Autodesk Inventor part; units mm, degrees
ref_plane "YZ Plane" through (0, 0, 0) normal (1, 0, 0) x (0, 1, 0)
ref_plane "XZ Plane" through (0, 0, 0) normal (0, 1, 0) x (-1, 0, 0)
ref_plane "XY Plane" through (0, 0, 0) normal (0, 0, 1) x (1, 0, 0)
sketch "Sketch1" plane through (0, 0, 0) normal (0, 0, 1) x (1, 0, 0)
  circle A0 centre (0, 0) radius 203.2
  dimension "d0" = 406.4
extrude "Extrusion1" add sketch "Sketch1" along normal blind 50.8
sketch "Sketch2" plane through (0, 0, 0) normal (1, 0, 0) x (0, 1, 0)
  circle A0 centre (-285.75, 25.4) radius 88.9
  line L0 (203.2, 0) -> (-203.2, 0)
  line L1 (0, 149.86) -> (0, -99.06)
  point P0 (0, 0)
  dimension "d3" = 25.4
  dimension "d4" = 177.8
  dimension "d5" = 285.75
revolve "Revolution1" cut sketch "Sketch2" angle 360 about axis through (0, 0, 0) along (0, 0, -1)
sketch "Sketch3" plane through (0, 0, 0) normal (0, 0, -1) x (-1, 0, 0)
  point P0 (0, 0)
sketch "Sketch4" plane through (0, 0, 50.8) normal (0, 0, 1) x (1, 0, 0)
  line L0 (-3.6662, 6.35) -> (3.6662, 6.35)
  line L1 (3.6662, 6.35) -> (7.3323, 0)
  line L2 (7.3323, 0) -> (3.6662, -6.35)
  line L3 (3.6662, -6.35) -> (-3.6662, -6.35)
  line L4 (-3.6662, -6.35) -> (-7.3323, 0)
  line L5 (-7.3323, 0) -> (-3.6662, 6.35)
  circle A0 centre (0, 23.8125) radius 2.5797
  circle A1 centre (-11.9062, 20.6222) radius 2.5797
  circle A2 centre (-20.6222, 11.9063) radius 2.5797
  circle A3 centre (-23.8125, 0) radius 2.5797
  circle A4 centre (-20.6222, -11.9062) radius 2.5797
  circle A5 centre (-11.9063, -20.6222) radius 2.5797
  circle A6 centre (0, -23.8125) radius 2.5797
  circle A7 centre (11.9062, -20.6222) radius 2.5797
  circle A8 centre (20.6222, -11.9063) radius 2.5797
  circle A9 centre (23.8125, 0) radius 2.5797
  circle A10 centre (20.6222, 11.9062) radius 2.5797
  circle A11 centre (11.9063, 20.6222) radius 2.5797
  point P0 (0, 0)
  point P1 (0, 0)
  dimension "d7" = 12.7
  dimension "d8" = 23.8125
  dimension "d9" = 5.1594
  dimension "d12" = 360
extrude "Extrusion2" cut sketch "Sketch4" against normal through all
sketch "Sketch6" plane through (0, 0, 0) normal (0, 0, -1) x (-1, 0, 0)
  circle A0 centre (0, 107.95) radius 2.5797
  circle A1 centre (0, 120.269) radius 4.445
  circle A2 centre (-41.3107, 99.7328) radius 2.5797
  circle A3 centre (-46.025, 111.1141) radius 4.445
  circle A4 centre (-76.3322, 76.3322) radius 2.5797
  circle A5 centre (-85.043, 85.043) radius 4.445
  circle A6 centre (-99.7328, 41.3107) radius 2.5797
  circle A7 centre (-111.1141, 46.025) radius 4.445
  circle A8 centre (-107.95, 0) radius 2.5797
  circle A9 centre (-120.269, 0) radius 4.445
  circle A10 centre (-99.7328, -41.3107) radius 2.5797
  circle A11 centre (-111.1141, -46.025) radius 4.445
  circle A12 centre (-76.3322, -76.3322) radius 2.5797
  circle A13 centre (-85.043, -85.043) radius 4.445
  circle A14 centre (-41.3107, -99.7328) radius 2.5797
  circle A15 centre (-46.025, -111.1141) radius 4.445
  circle A16 centre (0, -107.95) radius 2.5797
  circle A17 centre (0, -120.269) radius 4.445
  circle A18 centre (41.3107, -99.7328) radius 2.5797
  circle A19 centre (46.025, -111.1141) radius 4.445
  circle A20 centre (76.3322, -76.3322) radius 2.5797
  circle A21 centre (85.043, -85.043) radius 4.445
  circle A22 centre (99.7328, -41.3107) radius 2.5797
  circle A23 centre (111.1141, -46.025) radius 4.445
  circle A24 centre (107.95, 0) radius 2.5797
  circle A25 centre (120.269, 0) radius 4.445
  circle A26 centre (99.7328, 41.3107) radius 2.5797
  circle A27 centre (111.1141, 46.025) radius 4.445
  circle A28 centre (76.3322, 76.3322) radius 2.5797
  circle A29 centre (85.043, 85.043) radius 4.445
  circle A30 centre (41.3107, 99.7328) radius 2.5797
  circle A31 centre (46.025, 111.1141) radius 4.445
  point P0 (0, 0)
  dimension "d16" = 5.1594
  dimension "d17" = 107.95
  dimension "d18" = 8.89
  dimension "d19" = 120.269
  dimension "d22" = 360
extrude "Extrusion3" cut sketch "Sketch6" against normal through all
sketch "Sketch7" plane through (0, 0, 50.8) normal (0, 0, 1) x (1, 0, 0)
  circle A0 centre (0, 63.4238) radius 2.032
  circle A1 centre (-44.8474, 44.8474) radius 2.032
  circle A2 centre (-63.4238, 0) radius 2.032
  circle A3 centre (-44.8474, -44.8474) radius 2.032
  circle A4 centre (0, -63.4238) radius 2.032
  circle A5 centre (44.8474, -44.8474) radius 2.032
  circle A6 centre (63.4238, 0) radius 2.032
  circle A7 centre (44.8474, 44.8474) radius 2.032
  line L0 (0, 63.4238) -> (0, 0) construction
  circle A8 centre (11.1717, 56.164) radius 2.032
  line L1 (11.1717, 56.164) -> (0, 0) construction
  circle A9 centre (24.2712, 58.596) radius 4.445
  line L2 (24.2712, 58.596) -> (0, 0) construction
  circle A10 centre (-24.2712, 58.596) radius 4.445
  circle A11 centre (-58.596, 24.2712) radius 4.445
  circle A12 centre (-58.596, -24.2712) radius 4.445
  circle A13 centre (-24.2712, -58.596) radius 4.445
  circle A14 centre (24.2712, -58.596) radius 4.445
  circle A15 centre (58.596, -24.2712) radius 4.445
  circle A16 centre (58.596, 24.2712) radius 4.445
  circle A17 centre (-31.8143, 47.6135) radius 2.032
  circle A18 centre (-56.164, 11.1717) radius 2.032
  circle A19 centre (-47.6135, -31.8143) radius 2.032
  circle A20 centre (-11.1717, -56.164) radius 2.032
  circle A21 centre (31.8143, -47.6135) radius 2.032
  circle A22 centre (56.164, -11.1717) radius 2.032
  circle A23 centre (47.6135, 31.8143) radius 2.032
  line L3 (31.8143, 47.6135) -> (0, 0) construction
  circle A24 centre (31.8143, 47.6135) radius 4.445
  circle A25 centre (-11.1717, 56.164) radius 4.445
  circle A26 centre (-47.6135, 31.8143) radius 4.445
  circle A27 centre (-56.164, -11.1717) radius 4.445
  circle A28 centre (-31.8143, -47.6135) radius 4.445
  circle A29 centre (11.1717, -56.164) radius 4.445
  circle A30 centre (47.6135, -31.8143) radius 4.445
  circle A31 centre (56.164, 11.1717) radius 4.445
  dimension "d26" = 4.064
  dimension "d27" = 63.4238
  dimension "d30" = 360
  dimension "d32" = 4.064
  dimension "d33" = 57.2643
  dimension "d34" = 11.25
  dimension "d35" = 8.89
  dimension "d36" = 22.5
  dimension "d39" = 360
  dimension "d43" = 360
  dimension "d45" = 33.75
  dimension "d48" = 360
extrude "Extrusion4" cut sketch "Sketch7" against normal through all
properties part number "CenterIndexerWheel"
The listing builds one solid part. Answer for the finished solid, in the listing's coordinates (mm). Give positions to 0.01 mm unless a question says otherwise; leave off trailing zeros.
Item 1: Find the intervals of material crossed by line 1 along X through (y, z) = (45.5, 48.5); line 2 along X through (y, z) = (74, 6.5); line 3 along X through (y, z) = (-57, 33), in increasing order.
Item 2: Section A-A, the plane z = 46 is taken. Count the separate pieces of the cut face and the enclosed holes in it, plus the area to 3 significant figures.
Item 3: Flat-ended cylindrical pins translate along their axes: P1, Ø3, axis at x = 105, z = 39, coming from the -Y side; P2, Ø10, axis at x = -85.043, y = 85.043, coming from the -Z side; P3, Ø1.5, axis at x = -52, z = 37, coming from the -Y side; P4, Ø12, axis at y = -81.5, z = 44.5, coming from the -X side. Find the tip coordinate at first contact, or state that the pin passes through.
Completed:
1. line 1: x = -194.66 to -115.53, -106.7 to -46.77, -42.92 to 27.9, 35.72 to 42.92, 46.77 to 106.7, 115.53 to 194.66
1. line 2: x = -184.6 to -77.43, -75.23 to 75.23, 77.43 to 184.6
1. line 3: x = -188.76 to -28.42, -20.12 to -13.02, -9.32 to 6.81, 15.54 to 20.12, 28.42 to 188.76
2. separate pieces: 1
2. enclosed holes: 77
2. area: 122,000 mm2
3. P1: stops at y = -168.71
3. P2: stops at z = 0
3. P3: stops at y = -190.87
3. P4: stops at x = -184.49
